Work out the finished part from the listing and answer in its coordinate system (mm). A direction names the side the tool comes from. Coordinates: 2 decimals unless noted, no trailing zeros. Write each loop counter-clockwise with the first axis right and the second up, starting at its lowest first coordinate (ties: lowest second). Pieces come first, ordered by that corner, then holes. Notation, with made-up numbers: (-20, -10.5) - (-5, -10.5) arc R21 ccw to (-5, 25.5) - close; hole circle Ø10 at (33.25, -17). An arc over 180 degrees is marked (long way). One line per item, written item: value.
```python
from build123d import *

# Parameters (mm, degrees)
BOSS_EXTRUDE1_DEPTH = 3
SKETCH2_W           = 79.051219732
SKETCH2_H           = 181.686841404
CUT_EXTRUDE1_DEPTH  = 94.52539762


with BuildPart() as part:
    # Sketch1 → Boss-Extrude1 (new body)
    with BuildSketch(Plane(origin=(0, 0, 0), x_dir=(1, 0, 0), z_dir=(0, 1, 0))):
        Polygon((40, 80), (40, 70), (43, 70), (43, 60), (40, 60), (40, 50), (43, 50), (43, 40), (40, 40), (40, 30), (43, 30), (43, 20), (40, 20), (40, 10), (43, 10), (43, 0), (40, 0), (40, -10), (43, -10), (43, -20), (40, -20), (40, -30), (43, -30), (43, -40), (40, -40), (40, -50), (43, -50), (43, -60), (40, -60), (40, -70), (43, -70), (43, -80), (40, -80), (30, -80), (30, -83), (20, -83), (20, -80), (10, -80), (10, -83), (0, -83), (0, -80), (-10, -80), (-10, -83), (-20, -83), (-20, -80), (-30, -80), (-30, -83), (-40, -83), (-40, -80), (-40, -70), (-43, -70), (-43, -60), (-40, -60), (-40, -50), (-43, -50), (-43, -40), (-40, -40), (-40, -30), (-43, -30), (-43, -20), (-40, -20), (-40, -10), (-43, -10), (-43, 0), (-40, 0), (-40, 10), (-43, 10), (-43, 20), (-40, 20), (-40, 30), (-43, 30), (-43, 40), (-40, 40), (-40, 50), (-43, 50), (-43, 60), (-40, 60), (-40, 70), (-43, 70), (-43, 80), (-40, 80), (-30, 80), (-30, 83), (-20, 83), (-20, 80), (-10, 80), (-10, 83), (0, 83), (0, 80), (10, 80), (10, 83), (20, 83), (20, 80), (30, 80), (30, 83), (40, 83), align=None)
    extrude(amount=BOSS_EXTRUDE1_DEPTH)

    # Sketch2 → Cut-Extrude1 (cut, through all)
    with BuildSketch(Plane(origin=(0, 3, 0), x_dir=(1, 0, 0), z_dir=(0, 1, 0))):
        with Locations((19.525609866, -1.45411583)):
            Rectangle(SKETCH2_W, SKETCH2_H)
    extrude(amount=-CUT_EXTRUDE1_DEPTH, mode=Mode.SUBTRACT)


solid = part.part
```
Item 1: Which of the six approach directions +Z, -Z, +X, -X, +Y, -Y give full straight-line access (tool end or side, diameter ignored) to faces 1 (the face through (-40, 1, 76)), 2 (the face through (-25, 1, 80)), 3 (the face through (-42, 1, -20))?
Evaluation:
face 1: +Z, -X, +Y, -Y
face 2: +Z, +X, +Y, -Y
face 3: -X, +Y, -Y
Item 2: Section A-A, the plane x = -22.25 is taken. Determine the outline of the cut face in (y, z), then the cut area to 3 significant figures.
Evaluation:
outline: (0, -83) - (3, -83) - (3, 80) - (0, 80) - close
area: 489 mm2
Item 3: Consider probe 1 along Z at (x, y) = (-23, 1.8); probe 2 along X at (y, z) = (0.4, 19.5); probe 3 along Z at (x, y) = (-38, 1.2). Determine where each line is inside the solid, lowest interval first.
Evaluation:
probe 1: z = -83 to 80
probe 2: x = -40 to -20
probe 3: z = -80 to 83
Item 4: Determine the mould class of faces 4 (the face through (-43, 1, 5)), 5 (the face through (-41, 1, 70)), 6 (the face through (-41, 1, 10)) for opening direction Z: +Z half, -Z half, draft (parallel to the pull), parting line (faces both ways), or undercut.
Evaluation:
face 4: draft
face 5: +Z half
face 6: undercut
Item 5: Given pin 1 (1.5 mm diameter, centred on y = 1.5, z = -4.5, fed in from -X); pin 2 (1.5 mm diameter, centred on x = -39, y = 1, fed in from -Z); pin 3 (1.5 mm diameter, centred on y = 2, z = -81.5, fed in from -X), each flat-ended and moving along its own axis, determine where each tip first touches the part or whether it passes through.
Evaluation:
pin 1: stops at x = -40
pin 2: stops at z = -80
pin 3: stops at x = -30
